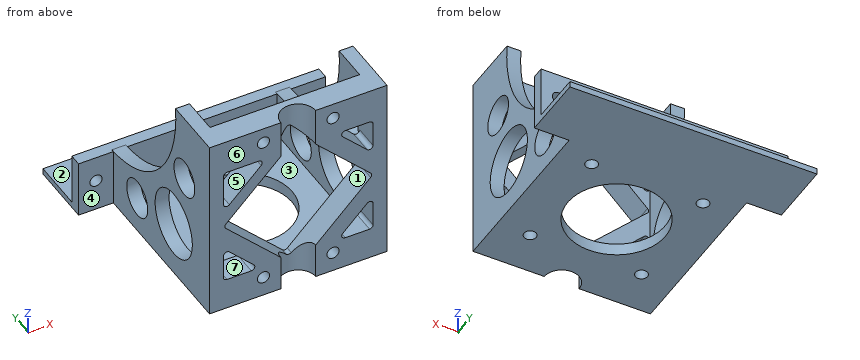
from build123d import *

# Parameters (mm, degrees)
SKETCH1_W                = 51
SKETCH1_H                = 53.5
BOSS_EXTRUDE1_DEPTH      = 54.25
SKETCH2_W                = 43
SKETCH2_H                = 43
CUT_EXTRUDE1_DEPTH       = 50.75
SKETCH3_W                = 43
SKETCH3_H                = 3.5
CUT_EXTRUDE2_DEPTH       = 37.5
CUT_EXTRUDE3_DEPTH       = 76
SKETCH5_R                = 9.673114497
SKETCH5_R_2              = 5.390775308
SKETCH5_R_3              = 5.456912487
CUT_EXTRUDE4_DEPTH       = 76
SKETCH6_R                = 14
SKETCH6_R_2              = 1.75
CUT_EXTRUDE5_DEPTH       = 76
SKETCH7_R                = 5
CUT_EXTRUDE6_DEPTH       = 76
CUT_EXTRUDE7_DEPTH       = 27
FILLET2_R                = 1
SKETCH12_R               = 1.75
CUT_EXTRUDE8_DEPTH       = 15
BOSS_EXTRUDE4_DEPTH      = 10
BOSS_EXTRUDE4_DEPTH_BACK = 61
SKETCH13_W               = 16.75
SKETCH13_H               = 3.5
SKETCH14_W               = 71
SKETCH14_H               = 1.75
BOSS_EXTRUDE5_DEPTH      = 15
SKETCH15_R               = 1.75
CUT_EXTRUDE9_DEPTH       = 10


with BuildPart() as part:
    # Sketch1 → Boss-Extrude1 (new body)
    with BuildSketch(Plane.XY):
        with Locations((-26.432354029, 2.021717979)):
            Rectangle(SKETCH1_W, SKETCH1_H)
    extrude(amount=BOSS_EXTRUDE1_DEPTH)

    # Sketch2 → Cut-Extrude1 (cut)
    with BuildSketch(Plane.XY.offset(54.25)):
        with Locations((-26.432354029, 3.771717979)):
            Rectangle(SKETCH2_W, SKETCH2_H)
    extrude(amount=-CUT_EXTRUDE1_DEPTH, mode=Mode.SUBTRACT)

    # Sketch3 → Cut-Extrude2 (cut)
    with BuildSketch(Plane.XY.offset(54.25)):
        with Locations((-26.432354029, 27.021717979)):
            Rectangle(SKETCH3_W, SKETCH3_H)
    extrude(amount=-CUT_EXTRUDE2_DEPTH, mode=Mode.SUBTRACT)

    # Sketch4 → Cut-Extrude3 (cut)
    with BuildSketch(Plane.ZY.offset(51.932354029)):
        with BuildLine():
            Line((16.75, 28.771717979), (54.25, 28.771717979))
            Line((54.25, 28.771717979), (54.25, -7.074674815))
            ThreePointArc((54.25, -7.074674815), (27.422353926, 2.398250742), (16.75, 28.771717979))
        make_face()
    extrude(amount=-CUT_EXTRUDE3_DEPTH, mode=Mode.SUBTRACT)

    # Sketch5 → Cut-Extrude4 (cut)
    with BuildSketch(Plane.ZY.offset(51.932354029)):
        with Locations(Location((15.954892055, -6.11697424, 0), (0, 0, 270))):
            Circle(SKETCH5_R)
        with Locations(Location((34.868290168, -11.652602956, 0), (0, 0, 270))):
            Circle(SKETCH5_R_2)
        with Locations(Location((10.551064023, 12.862324215, 0), (0, 0, 270))):
            Circle(SKETCH5_R_3)
    extrude(amount=-CUT_EXTRUDE4_DEPTH, mode=Mode.SUBTRACT)

    # Sketch6 → Cut-Extrude5 (cut)
    with BuildSketch(Plane.XY.offset(3.5)):
        with Locations((-26.432354029, 3.771717979)):
            Circle(SKETCH6_R)
        with Locations((-10.432354029, 19.771717979)):
            Circle(SKETCH6_R_2)
        with Locations((-42.432354029, 19.771717979)):
            Circle(SKETCH6_R_2)
        with Locations((-42.432354029, -12.228282021)):
            Circle(SKETCH6_R_2)
        with Locations((-10.432354029, -12.228282021)):
            Circle(SKETCH6_R_2)
    extrude(amount=-CUT_EXTRUDE5_DEPTH, mode=Mode.SUBTRACT)

    # Sketch7 → Cut-Extrude6 (cut)
    with BuildSketch(Plane(origin=(0, 0, 0), x_dir=(-1, 0, 0), z_dir=(0, 0, -1))):
        with Locations((26.432354029, -24.728282021)):
            Circle(SKETCH7_R)
    extrude(amount=-CUT_EXTRUDE6_DEPTH, mode=Mode.SUBTRACT)

    # Sketch8 → Cut-Extrude7 (cut)
    with BuildSketch(Plane.XZ.offset(24.728282021)):
        Polygon((-26.432354029, 48.25), (-4.932354029, 26.75), (-26.432354029, 5.25), (-47.932354029, 26.75), align=None)
        Polygon((-15.361286217, 44.25), (-4.932354029, 44.25), (-4.932354029, 33.821067812), align=None)
        Polygon((-4.932354029, 9.25), (-15.361286217, 9.25), (-4.932354029, 19.678932188), align=None)
        Polygon((-47.932354029, 9.25), (-37.503421841, 9.25), (-47.932354029, 19.678932188), align=None)
        Polygon((-47.932354029, 44.25), (-35.382101497, 44.25), (-47.932354029, 31.699747468), align=None)
    extrude(amount=-CUT_EXTRUDE7_DEPTH, mode=Mode.SUBTRACT)

    # Fillet2
    # the kernel refuses this fillet: 1 mm, written as the material it adds along each edge
    with BuildSketch(Plane(origin=(-47.932354029, -24.728282021, 31.699747468), x_dir=(0, 0, 1), z_dir=(0, 1, 0)), Plane(origin=(-4.932354029, -24.728282021, 19.678932188), x_dir=(0, 0, -1), z_dir=(0, 1, 0))) as fillet2_piece_1:
        with BuildLine():
            CenterArc((FILLET2_R * 2.41421356237, FILLET2_R), FILLET2_R, 135, 135)
            Line((FILLET2_R * 1.70710678119, FILLET2_R * 1.70710678119), (0, 0))
            Line((0, 0), (FILLET2_R * 2.41421356237, 0))
        make_face()
    extrude(amount=7)
    with BuildSketch(Plane(origin=(-4.932354029, -24.728282021, 33.821067812), x_dir=(0, 0, 1), z_dir=(0, 1, 0)), Plane(origin=(-47.932354029, -24.728282021, 19.678932188), x_dir=(0, 0, -1), z_dir=(0, 1, 0)), Plane(origin=(-15.361286217, -24.728282021, 9.25), x_dir=(1, 0, 0), z_dir=(0, 1, 0)), Plane(origin=(-37.503421841, -24.728282021, 9.25), x_dir=(-0.7071067811865486, 0, 0.7071067811865465), z_dir=(0, 1, 0)), Plane(origin=(-35.382101497, -24.728282021, 44.25), x_dir=(-1, 0, 0), z_dir=(0, 1, 0)), Plane(origin=(-15.361286217, -24.728282021, 44.25), x_dir=(0.7071067811865479, 0, -0.7071067811865472), z_dir=(0, 1, 0))) as fillet2_piece_2:
        with BuildLine():
            CenterArc((FILLET2_R * 2.41421356237, -FILLET2_R), FILLET2_R, 90, 135)
            Line((FILLET2_R * 1.70710678119, -FILLET2_R * 1.70710678119), (0, 0))
            Line((0, 0), (FILLET2_R * 2.41421356237, 0))
        make_face()
    extrude(amount=7)
    with BuildSketch(Plane(origin=(-26.432354029, -22.228282021, 5.25), x_dir=(0.7071067811865436, 0, 0.7071067811865516), z_dir=(0, 1, 0))) as fillet2_piece_3_section:
        with BuildLine():
            CenterArc((FILLET2_R, -FILLET2_R), FILLET2_R, 90, 90)
            Line((0, -FILLET2_R), (0, 0))
            Line((0, 0), (FILLET2_R, 0))
        make_face()
    fillet2_piece_3 = extrude(amount=4.5, mode=Mode.PRIVATE)
    fillet2_piece_3 = fillet2_piece_3 - Plane(origin=(-26.432354029, -24.728282021, 5.570701766), x_dir=(-1, 0, 0), z_dir=(0, 0, -1)) * Cylinder(5, 14, mode=Mode.PRIVATE)
    add(fillet2_piece_3)
    with BuildSketch(Plane(origin=(-4.932354029, -24.728282021, 9.25), x_dir=(0, 0, 1), z_dir=(0, 1, 0)), Plane(origin=(-47.932354029, -24.728282021, 26.75), x_dir=(0.7071067811865476, 0, -0.7071067811865476), z_dir=(0, 1, 0)), Plane(origin=(-47.932354029, -24.728282021, 44.25), x_dir=(0, 0, -1), z_dir=(0, 1, 0))) as fillet2_piece_4:
        with BuildLine():
            CenterArc((FILLET2_R, -FILLET2_R), FILLET2_R, 90, 90)
            Line((0, -FILLET2_R), (0, 0))
            Line((0, 0), (FILLET2_R, 0))
        make_face()
    extrude(amount=7)
    with BuildSketch(Plane(origin=(-47.932354029, -24.728282021, 9.25), x_dir=(0, 0, 1), z_dir=(0, 1, 0)), Plane(origin=(-4.932354029, -24.728282021, 26.75), x_dir=(-0.707106781186544, 0, -0.7071067811865511), z_dir=(0, 1, 0)), Plane(origin=(-4.932354029, -24.728282021, 44.25), x_dir=(0, 0, -1), z_dir=(0, 1, 0))) as fillet2_piece_5:
        with BuildLine():
            CenterArc((FILLET2_R, FILLET2_R), FILLET2_R, 180, 90)
            Line((0, FILLET2_R), (0, 0))
            Line((0, 0), (FILLET2_R, 0))
        make_face()
    extrude(amount=7)
    with BuildSketch(Plane(origin=(-26.432354029, -22.228282021, 48.25), x_dir=(0.7071067811865476, 0, -0.7071067811865476), z_dir=(0, 1, 0))) as fillet2_piece_6_section:
        with BuildLine():
            CenterArc((FILLET2_R, FILLET2_R), FILLET2_R, 180, 90)
            Line((0, FILLET2_R), (0, 0))
            Line((0, 0), (FILLET2_R, 0))
        make_face()
    fillet2_piece_6 = extrude(amount=4.5, mode=Mode.PRIVATE)
    fillet2_piece_6 = fillet2_piece_6 - Plane(origin=(-26.432354029, -24.728282021, 47.9292983), x_dir=(-1, 0, 0), z_dir=(0, 0, -1)) * Cylinder(5, 14, mode=Mode.PRIVATE)
    add(fillet2_piece_6)

    # Sketch12 → Cut-Extrude8 (cut)
    with BuildSketch(Plane.XZ.offset(24.728282021)):
        with Locations(Location((-16.432354029, 49.75, 0), (0, 0, 270))):
            Circle(SKETCH12_R)
        with Locations(Location((-36.432354029, 49.75, 0), (0, 0, 270))):
            Circle(SKETCH12_R)
        with Locations(Location((-16.432354029, 5.75, 0), (0, 0, 270))):
            Circle(SKETCH12_R)
        with Locations(Location((-36.432354029, 5.75, 0), (0, 0, 270))):
            Circle(SKETCH12_R)
    extrude(amount=-CUT_EXTRUDE8_DEPTH, mode=Mode.SUBTRACT)

    # Sketch13 → Boss-Extrude4 (add, two sides: drawn at the far end of the back side and taken through both)
    with BuildSketch(Plane.ZY.offset(51.932354029).offset(-BOSS_EXTRUDE4_DEPTH_BACK)):
        with Locations((8.375, 27.021717979)):
            Rectangle(SKETCH13_W, SKETCH13_H)
    extrude(amount=BOSS_EXTRUDE4_DEPTH + BOSS_EXTRUDE4_DEPTH_BACK)

    # Sketch14 → Boss-Extrude5 (add)
    with BuildSketch(Plane(origin=(0, 28.771717979, 0), x_dir=(1, 0, 0), z_dir=(0, 1, 0))):
        with Locations((-26.432354029, -0.875)):
            Rectangle(SKETCH14_W, SKETCH14_H)
    extrude(amount=BOSS_EXTRUDE5_DEPTH)

    # Sketch15 → Cut-Extrude9 (cut)
    with BuildSketch(Plane.XZ.offset(-25.271717979)):
        with Locations((-56.932354029, 9.25)):
            Circle(SKETCH15_R)
        with Locations((4.067645971, 9.25)):
            Circle(SKETCH15_R)
    extrude(amount=-CUT_EXTRUDE9_DEPTH, mode=Mode.SUBTRACT)


solid = part.part
Can you work these out from the model? Positions are in its coordinate system, mm. Face numbers are marked on the shaded views. A direction names the side the tool comes from. Coordinates: 2 decimals unless noted, no trailing zeros. Order: outer loops, then holes, each group sorted by start corner. A loop starts at its lowest first (then second) coordinate and runs counter-clockwise, first axis right, second up. Notation, with made-up numbers: (-36.75, 84) -> (-5.75, 84) arc R18 cw to (-5.75, 111) -> close; hole circle Ø10 at (13, 62). An arc over 180 degrees is marked (long way). Use one line per item in the form item = value.
Q1. Imagine slicing it at B-B, the plane y = 5.5. List the corners of the cut face in (x, z) for me.
From the geometry:
outline = (-51.93, 0) -> (-40.33, 0) -> (-40.33, 3.5) -> (-47.93, 3.5) -> (-47.93, 24.55) -> (-51.93, 24.55) -> close; (-12.54, 0) -> (-0.93, 0) -> (-0.93, 24.55) -> (-4.93, 24.55) -> (-4.93, 3.5) -> (-12.54, 3.5) -> close
Q2. Which directions (+Z, -Z, +X, -X, +Y, -Y) give clear straight access to the entire face, cutting with the end or side of a thin tool? Please do the marked faces 1, 2, 3, 4 and 5.
From the geometry:
face_1 = -Y
face_2 = +Z, +X, -X, +Y
face_3 = +Z
face_4 = +Z, -Z, -X, -Y
face_5 = +Y, -Y
Q3. Imagine slicing it at C-C, the plane z = 38.5. List the corners of the cut face in (x, y) for me, then the cut area to 3 significant figures.
From the geometry:
outline = (-51.93, -24.73) -> (-47.93, -24.73) -> (-47.93, -15.64) -> (-51.93, -15.64) -> close; (-51.93, -7.67) -> (-47.93, -7.67) -> (-47.93, -4.73) -> (-51.93, -4.73) -> close; (-41.13, -24.73) -> (-36.18, -24.73) -> (-36.18, -17.73) -> (-41.13, -17.73) -> close; (-16.68, -24.73) -> (-9.61, -24.73) -> (-9.61, -17.73) -> (-16.68, -17.73) -> close; (-4.93, -24.73) -> (-0.93, -24.73) -> (-0.93, -15.64) -> (-4.93, -15.64) -> close; (-4.93, -7.67) -> (-0.93, -7.67) -> (-0.93, -4.73) -> (-4.93, -4.73) -> close
area = 180 mm²
Q4. Imagine slicing it at A-A, the plane z = 50.5. List the corners of the cut face in (x, y) for me, then the cut area to 3 significant figures.
From the geometry:
outline = (-51.93, -24.73) -> (-38.01, -24.73) -> (-38.01, -17.73) -> (-47.93, -17.73) -> (-47.93, -7.19) -> (-51.93, -7.19) -> close; (-34.85, -24.73) -> (-31.43, -24.73) arc R5 cw to (-21.43, -24.73) -> (-18.01, -24.73) -> (-18.01, -17.73) -> (-34.85, -17.73) -> close; (-14.85, -24.73) -> (-0.93, -24.73) -> (-0.93, -7.19) -> (-4.93, -7.19) -> (-4.93, -17.73) -> (-14.85, -17.73) -> close
area = 358 mm²
Q5. Will these pins go through, and if not, where does the flat tip stop? P1, Ø16.5, axis at x = -18.5, z = 12.5, coming from the +Y side; P2, Ø5, axis at x = -59, z = 10, coming from the -Y side; P3, Ø12, axis at x = -29, y = 33.5, coming from the +Z side.
From the geometry:
P1 = 28.77
P2 = 25.27
P3 = 16.75
Q6. We'd pull the mould along X, two halves only. Please class the marked faces 6 and 7: released by +X, released by -X, zero draft, split by the parting line, or undercut.
From the geometry:
face_6 = zero draft
face_7 = undercut
Q7. Imagine slicing it at D-D, the plane z = 23. List the corners of the cut face in (x, y) for me, then the cut area to 3 significant figures.
From the geometry:
outline = (-51.93, -24.73) -> (-44.18, -24.73) -> (-44.18, -17.73) -> (-47.93, -17.73) -> (-47.93, -12.75) -> (-51.93, -12.75) -> close; (-51.93, 0.51) -> (-47.93, 0.51) -> (-47.93, 7.55) -> (-51.93, 7.55) -> close; (-8.68, -24.73) -> (-0.93, -24.73) -> (-0.93, -12.75) -> (-4.93, -12.75) -> (-4.93, -17.73) -> (-8.68, -17.73) -> close; (-4.93, 0.51) -> (-0.93, 0.51) -> (-0.93, 7.55) -> (-4.93, 7.55) -> close
area = 205 mm²
Q8. I need wall thicknesses on L1, parallel to X at y = 26, z = 9; L2, parallel to X at y = -11.5, z = 46.5; L3, parallel to Y at x = -38, z = 8.5. Which ranges of each line are inside material? Lowest first, please.
From the geometry:
L1 = -61.93 to -58.66, -55.2 to 2.34, 5.8 to 9.07
L2 = -51.93 to -47.93, -4.93 to -0.93
L3 = -24.73 to -17.73, 25.27 to 28.77
